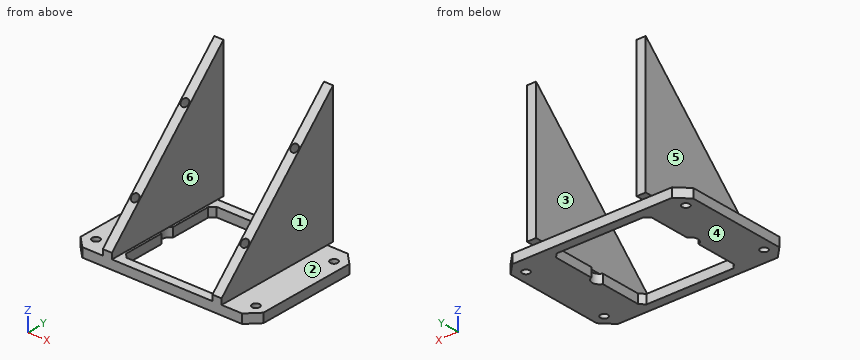
from build123d import *

# Parameters (mm, degrees)
F_4MM_START                  = 7
SKETCH_1_R                   = 1.65
F_4MM_DEPTH                  = 4
EXTRUDE_START                = -26
EXTRUDE_45_1_DEPTH           = 4
EXTRUDE_START_2              = 22
EXTRUDE_45_1_2_DEPTH         = 4
CUT_EXTRUDE_48X36_DEPTH      = 14
CUT_EXTRUDE_48X36_DEPTH_BACK = 14
SKETCH_4_R                   = 1.65
CUT_EXTRUDE_START            = 7
SKETCH_5_R                   = 3.1
CUT_EXTRUDE_631_DEPTH        = 4


with BuildPart() as part:
    # Sketch 1 → 4mm (new body)
    with BuildSketch(Plane.XY.offset(F_4MM_START)):
        Polygon((-35, -112), (35, -112), (40, -107), (40, -63), (35, -58), (-35, -58), (-40, -63), (-40, -107), align=None)
        with Locations((-35, -105)):
            Circle(SKETCH_1_R, mode=Mode.SUBTRACT)
        with Locations((-35, -65)):
            Circle(SKETCH_1_R, mode=Mode.SUBTRACT)
        with Locations((35, -105)):
            Circle(SKETCH_1_R, mode=Mode.SUBTRACT)
        with Locations((35, -65)):
            Circle(SKETCH_1_R, mode=Mode.SUBTRACT)
        Polygon((-19, -108), (19, -108), (21, -106), (21, -64), (19, -62), (-19, -62), (-21, -64), (-21, -106), align=None, mode=Mode.SUBTRACT)
    extrude(amount=F_4MM_DEPTH)

    # Sketch 2 → Extrude 45__-1 (add)
    with BuildSketch(Plane(origin=(0, 0, 0), x_dir=(0, 0, -1), z_dir=(1, 0, 0)).offset(EXTRUDE_START)):
        Polygon((-11, -112), (-11, -55), (-70.5, -55), (-13.5, -112), align=None)
    extrude(amount=EXTRUDE_45_1_DEPTH)

    # Sketch 3 → Extrude 45__1 2 (add)
    with BuildSketch(Plane(origin=(0, 0, 0), x_dir=(0, 0, -1), z_dir=(1, 0, 0)).offset(EXTRUDE_START_2)):
        Polygon((-11, -112), (-11, -55), (-70.5, -55), (-13.5, -112), align=None)
    extrude(amount=EXTRUDE_45_1_2_DEPTH)

    # Sketch 4 → Cut-Extrude 48x36 (cut, two sides: drawn at the far end of the back side and taken through both)
    with BuildSketch(Plane(origin=(0, -62.75, 62.75), x_dir=(1, 0, 0), z_dir=(0, -0.7071067811865475, 0.7071067811865476)).offset(-CUT_EXTRUDE_48X36_DEPTH_BACK)):
        with Locations(Location((-24, -49.539844892, 0), (0, 0, 270))):
            Circle(SKETCH_4_R)
        with Locations(Location((-24, -13.539844892, 0), (0, 0, 270))):
            Circle(SKETCH_4_R)
        with Locations(Location((24, -49.539844892, 0), (0, 0, 270))):
            Circle(SKETCH_4_R)
        with Locations(Location((24, -13.539844892, 0), (0, 0, 270))):
            Circle(SKETCH_4_R)
    extrude(amount=CUT_EXTRUDE_48X36_DEPTH + CUT_EXTRUDE_48X36_DEPTH_BACK, mode=Mode.SUBTRACT)

    # Sketch 5 → Cut-Extrude 631 (cut)
    with BuildSketch(Plane.XY.offset(CUT_EXTRUDE_START)):
        with Locations((-20, -85)):
            Circle(SKETCH_5_R)
        with Locations((20, -85)):
            Circle(SKETCH_5_R)
    extrude(amount=CUT_EXTRUDE_631_DEPTH, mode=Mode.SUBTRACT)


solid = part.part
Geometry check sheet. Reference: the model listing, model coordinates, mm. Face numbers are marked on the shaded views. A direction names the side the tool comes from. Give positions to 0.01 mm unless a question says otherwise; leave off trailing zeros. Loops run counter-clockwise (first coordinate to the right, second up) from the corner with the lowest first, then second, coordinate; pieces in that order, holes last. Notation, with made-up numbers: (48, -14.75) -> (59, -14.75) arc R19 cw to (59, 6.25) -> close; hole circle Ø3 at (32.25, 10). An arc over 180 degrees is marked (long way). Answer in a Markdown table with one row per item. Add a question column.
1) Cross-section at C-C on y = -105. Record the boundary of the cut face in (x, z).
2) Gauge pin test, flat ends, axial feed: P1, Ø10, axis at x = -23.5, y = -100.5, coming from the +Z side; P2, Ø4, axis at x = -35, y = -105, coming from the +Z side; P3, Ø3, axis at y = -74, z = 14, coming from the +X side. Record the tip position at first contact, or that the pin passes through.
3) Draft check along X on the marked faces 1, 2 and 3. Enter one of: pulls with the +X half, pulls with the -X half, needs draft (parallel to the pull), parting line crosses it, or undercut.
4) Material ranges on probe 1 along X at (y, z) = (-65, 9); probe 2 along Y at (x, z) = (-35, 9); probe 3 along X at (y, z) = (-85, 18), recorded low to high. Write a range as from..to.
5) Cross-section at B-B on x = 15. Record the boundary of the cut face in (y, z), and give its area (3 significant figures).
6) Cross-section at D-D on y = -79. Record the boundary of the cut face in (x, z).
7) Set-up check for the marked faces 4, 5 and 6: record each of +Z, -Z, +X, -X, +Y, -Y from which the full face is reachable in a straight line by a thin tool's end or side.
8) Cross-section at A-A on z = 15.5. Record the boundary of the cut face in (x, y), and give its area (3 significant figures).
Outcome:
| question | item | result |
|---|---|---|
| 1 | outline | (-40, 7) -> (-36.65, 7) -> (-36.65, 11) -> (-40, 11) -> close; (-33.35, 7) -> (-21, 7) -> (-21, 11) -> (-22, 11) -> (-22, 20.5) -> (-26, 20.5) -> (-26, 11) -> (-33.35, 11) -> close; (21, 7) -> (33.35, 7) -> (33.35, 11) -> (26, 11) -> (26, 20.5) -> (22, 20.5) -> (22, 11) -> (21, 11) -> close; (36.65, 7) -> (40, 7) -> (40, 11) -> (36.65, 11) -> close |
| 2 | P1 | stops at z = 30 |
| 2 | P2 | stops at z = 11 |
| 2 | P3 | stops at x = 26 |
| 3 | face 1 | pulls with the +X half |
| 3 | face 2 | needs draft |
| 3 | face 3 | undercut |
| 4 | probe 1 | x = -40..-36.65, -33.35..-21, 21..33.35, 36.65..40 |
| 4 | probe 2 | y = -112..-106.65, -103.35..-66.65, -63.35..-58 |
| 4 | probe 3 | x = -26..-22, 22..26 |
| 5 | outline | (-112, 7) -> (-108, 7) -> (-108, 11) -> (-112, 11) -> close; (-62, 7) -> (-58, 7) -> (-58, 11) -> (-62, 11) -> close |
| 5 | area | 32.0 mm^2 |
| 6 | outline | (-40, 7) -> (-21, 7) -> (-21, 11) -> (-22, 11) -> (-22, 46.5) -> (-26, 46.5) -> (-26, 11) -> (-40, 11) -> close; (21, 7) -> (40, 7) -> (40, 11) -> (26, 11) -> (26, 46.5) -> (22, 46.5) -> (22, 11) -> (21, 11) -> close |
| 7 | face 4 | -Z, +X, -X, +Y, -Y |
| 7 | face 5 | +Z, -X, +Y, -Y |
| 7 | face 6 | +Z, +Y, -Y |
| 8 | outline | (-26, -110) -> (-22, -110) -> (-22, -55) -> (-26, -55) -> close; (22, -110) -> (26, -110) -> (26, -55) -> (22, -55) -> close |
| 8 | area | 440 mm^2 |
